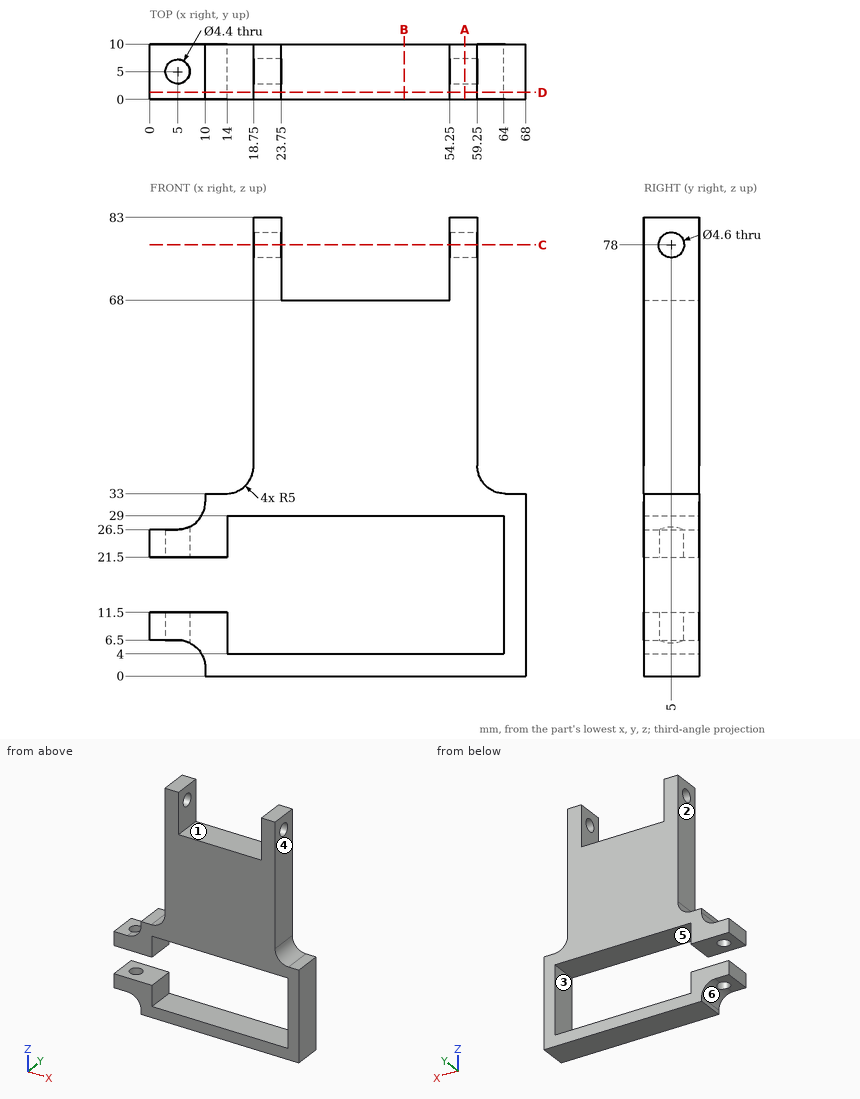
Input: dimensioned drawing with shaded views. Units: mm. Origin: part minimum x, y, z. A direction names the side the tool comes from. Round coordinates to 2 decimals unless told otherwise and drop trailing zeros. Order: outer loops, then holes, each group sorted by start corner. A loop starts at its lowest first (then second) coordinate and runs counter-clockwise, first axis right, second up. Notation, with made-up numbers: (-20.75, -2.5) -> (-7.75, -2.5) arc R16 ccw to (-7.75, 4.5) -> close; hole circle Ø1 at (-17, -11.5). An arc over 180 degrees is marked (long way). Put each result on its own line as item: value. Start each with the question number.
Q1. Line query: probe 1 along X at (y, z) = (5, 7.1); probe 2 along Z at (x, y) = (57.5, 2); probe 3 along Y at (x, z) = (5, 8). Output: solid intervals per line, ascending.
Q2. First-contact query: pin 1 (5 mm diameter, centred on y = 6, z = 50.5, fed in from -X); pin 2 (5 mm diameter, centred on x = 5, y = 5, fed in from -Z); pin 3 (2.5 mm diameter, centred on x = 3, y = 3.5, fed in from -Z); pin 4 (1.5 mm diameter, centred on x = 57, y = 6.5, fed in from -Z). Flat tips, straight axial feed; report the tip coordinate or a pass-through.
Q3. Section D-D on y = 1.25. Return the cut outline in (x, z).
Q4. Section C-C on z = 78. Return the cut outline in (x, y).
Q5. Pull-direction query (X, two-part tool) for the marked faces 4, 5 and 6; classes: +X half, -X half, draft (parallel to the pull), parting line (faces both ways), or undercut.
Q6. Section A-A on x = 57. Return the cut outline in (y, z).
Q7. Section B-B on x = 46. Return the cut outline in (y, z), and give its area (3 significant figures).
Q8. Reachability of the marked faces 1, 2 and 3 from +Z, -Z, +X, -X, +Y, -Y: full face, straight path, thin tool, end or side. Return the list, or none.
Ans:
1. probe 1: x = 0 to 2.8, 7.2 to 14, 64 to 68
1. probe 2: z = 0 to 4, 29 to 83
1. probe 3: y = 0 to 2.8, 7.2 to 10
2. pin 1: stops at x = 18.75
2. pin 2: stops at z = 5.83
2. pin 3: stops at z = 6.5
2. pin 4: stops at z = 0
3. outline: (0, 6.5) -> (5, 6.5) arc R5 cw to (10, 1.5) -> (10, 0) -> (68, 0) -> (68, 33) -> (64.25, 33) arc R5 cw to (59.25, 38) -> (59.25, 83) -> (54.25, 83) -> (54.25, 68) -> (23.75, 68) -> (23.75, 83) -> (18.75, 83) -> (18.75, 38) arc R5 cw to (13.75, 33) -> (10, 33) -> (10, 31.5) arc R5 cw to (5, 26.5) -> (0, 26.5) -> (0, 21.5) -> (14, 21.5) -> (14, 29) -> (64, 29) -> (64, 4) -> (14, 4) -> (14, 11.5) -> (0, 11.5) -> close
4. outline: (18.75, 0) -> (23.75, 0) -> (23.75, 2.7) -> (18.75, 2.7) -> close; (18.75, 7.3) -> (23.75, 7.3) -> (23.75, 10) -> (18.75, 10) -> close; (54.25, 0) -> (59.25, 0) -> (59.25, 2.7) -> (54.25, 2.7) -> close; (54.25, 7.3) -> (59.25, 7.3) -> (59.25, 10) -> (54.25, 10) -> close
5. face 4: +X half
5. face 5: undercut
5. face 6: -X half
6. outline: (0, 0) -> (10, 0) -> (10, 4) -> (0, 4) -> close; (0, 29) -> (10, 29) -> (10, 83) -> (0, 83) -> close; hole circle Ø4.6 at (5, 78)
7. outline: (0, 0) -> (10, 0) -> (10, 4) -> (0, 4) -> close; (0, 29) -> (10, 29) -> (10, 68) -> (0, 68) -> close
7. area: 430 mm2
8. face 1: +Z, +Y, -Y
8. face 2: +Z, -X, +Y, -Y
8. face 3: +Y, -Y
